Check sheet for the modelled part. Datum: model origin and axes. Units: mm. Face numbers are marked on the shaded views. A direction names the side the tool comes from. Round coordinates to 2 decimals unless told otherwise and drop trailing zeros. Loops run counter-clockwise (first coordinate to the right, second up) from the corner with the lowest first, then second, coordinate; pieces in that order, holes last. Notation, with made-up numbers: (61.25, -35.75) - (75.25, -35.75) arc R19 cw to (75.25, -2.75) - close; hole circle Ø9 at (-13, 30). An arc over 180 degrees is marked (long way). Answer in a Markdown table with one row per item. Add a question column.
(1) Gauge pin test, flat ends, axial feed: pin 1 (2 mm diameter, centred on y = -1.5, z = 2, fed in from +X); pin 2 (8 mm diameter, centred on x = 0, y = 0, fed in from -Z); pin 3 (1.5 mm diameter, centred on y = 10, z = -2.5, fed in from +X). Record the tip position at first contact, or that the pin passes through.
(2) Thickness scan on line 1 along Y through (x, z) = (0, 0.2); line 2 along Y through (x, z) = (0, 1.05); line 3 along Z through (x, y) = (-2.5, 8.5). Record the ranges inside material, lowest first.
(3) Access from +Z, -Z, +X, -X, +Y, -Y to the whole of each face (thin tool, end or side, straight path). Record for the marked faces 3 and 4.
(4) Cross-section at A-A on x = 0. Enter the section's corners in (y, z).
(5) Mould release check, pull along X, two halves, no side actions. Record for the marked faces 1 and 2: +X half, -X half, draft (parallel to the pull), parting line (faces both ways), or undercut.
(6) Cross-section at C-C on z = 2. Enter the section's corners in (x, y), then the cut area to 3 significant figures.
from build123d import *


with BuildPart() as f1:
    # F0 (on Front) → F1 (revolve)
    with BuildSketch(Plane.XZ):
        with BuildLine():
            ThreePointArc((11.070714, -3.5), (12.128908, -1.890295), (12.5, 0))
            ThreePointArc((12.5, 0), (12.128908, 1.890295), (11.070714, 3.5))
            Line((11.070714, 3.5), (9.070714, 3.5))
            Line((9.070714, 3.5), (9.070714, 2.5))
            Line((9.070714, 2.5), (2.5, 2.5))
            Line((2.5, 2.5), (2.5, 0))
            Line((2.5, 0), (2.5, -2.5))
            Line((2.5, -2.5), (9.070714, -2.5))
            Line((9.070714, -2.5), (9.070714, -3.5))
            Line((9.070714, -3.5), (11.070714, -3.5))
        make_face()
    revolve(axis=Axis((0, 0, 4.247276), (0, 0, 1)))


solid = f1.part
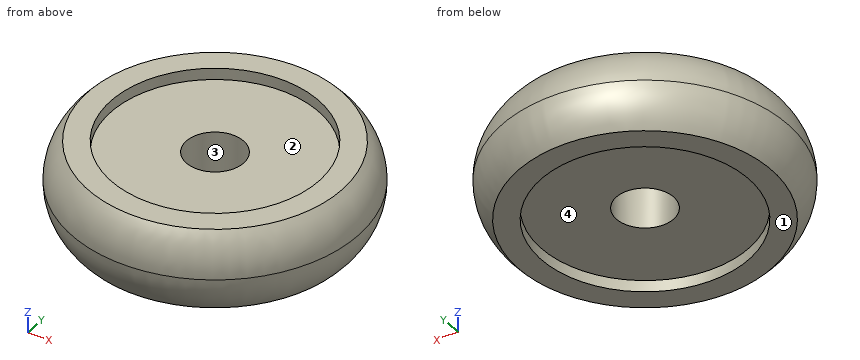
Answers:
| question | item | result |
|---|---|---|
| 1 | pin 1 | stops at x = 12.33 |
| 1 | pin 2 | stops at z = -2.5 |
| 1 | pin 3 | stops at x = 7.56 |
| 2 | line 1 | y = -12.5 to -2.5, 2.5 to 12.5 |
| 2 | line 2 | y = -12.39 to -2.5, 2.5 to 12.39 |
| 2 | line 3 | z = -2.5 to 2.5 |
| 3 | face 3 | +Z, -Z |
| 3 | face 4 | -Z |
| 4 | outline | (-12.5, 0) arc R5 ccw to (-11.07, -3.5) - (-9.07, -3.5) - (-9.07, -2.5) - (-2.5, -2.5) - (-2.5, 2.5) - (-9.07, 2.5) - (-9.07, 3.5) - (-11.07, 3.5) arc R5 ccw to start; (2.5, -2.5) - (9.07, -2.5) - (9.07, -3.5) - (11.07, -3.5) arc R5 ccw to (12.5, 0) arc R5 ccw to (11.07, 3.5) - (9.07, 3.5) - (9.07, 2.5) - (2.5, 2.5) - close |
| 5 | face 1 | draft |
| 5 | face 2 | undercut |
| 6 | outline | circle Ø24.17 at (0, 0); hole circle Ø5 at (0, 0) |
| 6 | area | 439 mm^2 |
